For this review, take the finished solid that the model builds, in its own axes (mm). Round coordinates to 2 decimals unless told otherwise and drop trailing zeros. Write each loop counter-clockwise with the first axis right and the second up, starting at its lowest first coordinate (ties: lowest second). Pieces come first, ordered by that corner, then holes. Notation, with made-up numbers: M 85.25,33.5 L 140.25,33.5 A25 cw 140.25,66.5 Z; hole C 71.25,-26 d4. An arc over 180 degrees is marked long. Answer in a Markdown table with one row per item.
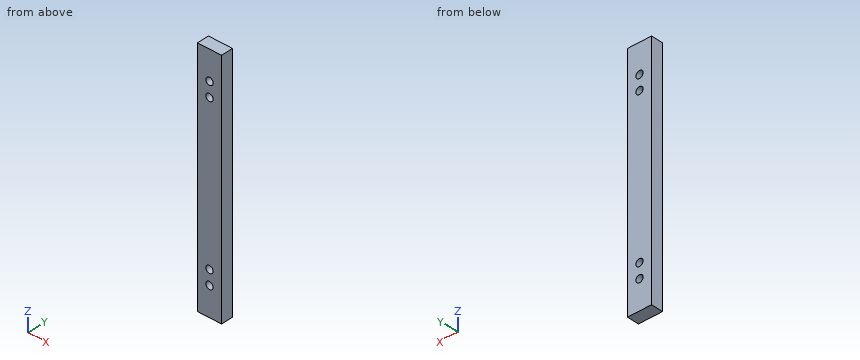
Autodesk Inventor part; units mm, degrees
ref_plane "YZ Plane" through (0, 0, 0) normal (1, 0, 0) x (0, 1, 0)
ref_plane "XZ Plane" through (0, 0, 0) normal (0, 1, 0) x (-1, 0, 0)
ref_plane "XY Plane" through (0, 0, 0) normal (0, 0, 1) x (1, 0, 0)
sketch "Sketch1" plane through (0, 0, 0) normal (0, 1, 0) x (-1, 0, 0)
  line L0 (0, 0) -> (10, 0)
  line L1 (10, 0) -> (10, -100)
  line L2 (10, -100) -> (0, -100)
  line L3 (0, -100) -> (0, 0)
  dimension "d0" = 10
  dimension "d1" = 100
extrude "Extrusion1" add sketch "Sketch1" along normal blind 5
sketch "Sketch2" plane through (0, 5, 0) normal (0, 1, 0) x (1, 0, 0)
  circle A0 centre (-5, 12) radius 1.5
  line L0 (0, 0) -> (0, 100)
  line L1 (-10, 0) -> (0, 0)
  circle A1 centre (-5, 18) radius 1.5
  line L2 (0, 0) -> (0, 50)
  circle A2 centre (-5, 88) radius 1.5
  circle A3 centre (-5, 82) radius 1.5
  dimension "d4" = 3
  dimension "d8" = 5
  dimension "d9" = 12
  dimension "d12" = 3
  dimension "d13" = 6
  dimension "d14" = 0
  dimension "d15" = 50
extrude "Extrusion2" cut sketch "Sketch2" against normal through all
properties part number "Soporte2_Dos"
Q1. Take a section at B-B (y = 2.25). State the section outline as (x, z) points, then the cut area to 3 significant figures.
Found:
| item | result |
|---|---|
| outline | M -10,-100 L 0,-100 L 0,0 L -10,0 Z; hole C -5,-88 d3; hole C -5,-82 d3; hole C -5,-18 d3; hole C -5,-12 d3 |
| area | 972 mm² |
Q2. For probe 1 along Z at (x, y) = (-5, 2.5); probe 2 along X at (y, z) = (3.7, -88); probe 3 along Z at (x, y) = (-5.5, 1.05), list the stretches that pass through material, from the lowest coordinate up.
Found:
| item | result |
|---|---|
| probe 1 | -100 to -89.5, -86.5 to -83.5, -80.5 to -19.5, -16.5 to -13.5, -10.5 to 0 |
| probe 2 | -10 to -6.5, -3.5 to 0 |
| probe 3 | -100 to -89.41, -86.59 to -83.41, -80.59 to -19.41, -16.59 to -13.41, -10.59 to 0 |
Q3. Take a section at A-A (z = -12). State the section outline as (x, y) points, then the cut area to 3 significant figures.
Found:
| item | result |
|---|---|
| outline | M -10,0 L -6.5,0 L -6.5,5 L -10,5 Z; M -3.5,0 L 0,0 L 0,5 L -3.5,5 Z |
| area | 35.0 mm² |
Q4. Insertion check: P1, Ø2.5, axis at x = -5, z = -82, coming from the -Y side (3 decimals). The pin has a flat end and moves straight along its axis. Give the tip position at first contact, or say it passes through.
Found:
| item | result |
|---|---|
| P1 | through |
Q5. Take a section at C-C (x = -5). State the section outline as (y, z) points, then the cut area to 3 significant figures.
Found:
| item | result |
|---|---|
| outline | M 0,-100 L 5,-100 L 5,-89.5 L 0,-89.5 Z; M 0,-86.5 L 5,-86.5 L 5,-83.5 L 0,-83.5 Z; M 0,-80.5 L 5,-80.5 L 5,-19.5 L 0,-19.5 Z; M 0,-16.5 L 5,-16.5 L 5,-13.5 L 0,-13.5 Z; M 0,-10.5 L 5,-10.5 L 5,0 L 0,0 Z |
| area | 440 mm² |
